```python
from build123d import *

# Parameters (mm, degrees)
SKETCH_1_W          = 550
SKETCH_1_H          = 550
SKETCH_1_R          = 200
EXTRUDE_1_DEPTH     = 3
SKETCH_2_R          = 2
CUT_EXTRUDE_1_DEPTH = 389.920300319
CHAMFER_1_SIZE      = 2


with BuildPart() as part:
    # 草图1 → 凸台-拉伸1 (new body)
    with BuildSketch(Plane(origin=(0, 0, 0), x_dir=(1, 0, 0), z_dir=(0, 1, 0))):
        Rectangle(SKETCH_1_W, SKETCH_1_H)
        with Locations(Location((0, 0, 0), (0, 0, 270))):
            Circle(SKETCH_1_R, mode=Mode.SUBTRACT)
    extrude(amount=EXTRUDE_1_DEPTH)

    # 草图2 → 切除-拉伸1 (cut, through all)
    with BuildSketch(Plane(origin=(0, 0, 0), x_dir=(1, 0, 0), z_dir=(0, 1, 0))):
        with Locations(Location((-260, 260, 0), (0, 0, 270))):
            Circle(SKETCH_2_R)
        with Locations(Location((-100, 260, 0), (0, 0, 270))):
            Circle(SKETCH_2_R)
        with Locations(Location((100, 260, 0), (0, 0, 90))):
            Circle(SKETCH_2_R)
        with Locations(Location((260, -100, 0), (0, 0, 90))):
            Circle(SKETCH_2_R)
        with Locations(Location((260, 100, 0), (0, 0, 270))):
            Circle(SKETCH_2_R)
        with Locations(Location((260, 260, 0), (0, 0, 270))):
            Circle(SKETCH_2_R)
        with Locations(Location((-100, -260, 0), (0, 0, 90))):
            Circle(SKETCH_2_R)
        with Locations(Location((100, -260, 0), (0, 0, 270))):
            Circle(SKETCH_2_R)
        with Locations(Location((260, -260, 0), (0, 0, 270))):
            Circle(SKETCH_2_R)
        with Locations(Location((-260, 100, 0), (0, 0, 90))):
            Circle(SKETCH_2_R)
        with Locations(Location((-260, -100, 0), (0, 0, 270))):
            Circle(SKETCH_2_R)
        with Locations(Location((-260, -260, 0), (0, 0, 270))):
            Circle(SKETCH_2_R)
    extrude(amount=CUT_EXTRUDE_1_DEPTH, mode=Mode.SUBTRACT)

    # 倒角1
    chamfer_1_edges = [part.edges().sort_by_distance(p)[0] for p in [
        (-260, 3, -98),
        (-260, 3, 98),
        (-260, 3, 258),
        (-100, 3, 262),
        (100, 3, 258),
        (260, 3, 258),
        (260, 3, 102),
        (260, 3, -102),
        (260, 0, -262),
        (100, 3, -258),
        (-100, 3, -262),
        (-260, 3, -262),
    ]]
    chamfer(chamfer_1_edges, length=CHAMFER_1_SIZE)


solid = part.part
```
Source: CAD feature listing. Evaluate the final solid. Frame: model axes, mm. Give positions to 0.01 mm unless a question says otherwise; leave off trailing zeros. Loops run counter-clockwise (first coordinate to the right, second up) from the corner with the lowest first, then second, coordinate; pieces in that order, holes last. Notation, with made-up numbers: (27, 15) -> (80, 15) arc R21 ccw to (80, 22) -> close; hole circle Ø5 at (76, 28.5). An arc over 180 degrees is marked (long way). Put each result on its own line as item: value. Start each with the question number.
1) Draft query along X for faces 1 (the face through (118, 3, -187)), 2 (the face through (60.075, 1.479, 190.764)). Return one class per face: released by +X, released by -X, zero draft, split by the parting line, or undercut.
2) Contact query for flat-ended pins moving along their axis: P1, Ø5, axis at x = 260, z = 260, coming from the -Y side; P2, Ø3, axis at x = 100, z = 260, coming from the +Y side; P3, Ø4.5, axis at x = 100, z = -260, coming from the +Y side; P4, Ø6.5, axis at x = -100, z = -260, coming from the +Y side. Output: stop coordinate, or through.
3) Cut plane A-A (x = 0). Return loops of the section in (y, z), then the cut area to 3 significant figures.
4) Cut plane C-C (y = 0.45). State how many separate pieces and enclosed holes the cut face has, then the cut area to 3 significant figures.
5) Material intervals for probe 1 along Z at (x, y) = (-260, 0.3); probe 2 along X at (y, z) = (0.7, -260), sorted ascending.
6) Cut plane B-B (z = 0). Return loops of the section in (x, y).
Results are:
1. face 1: zero draft
1. face 2: undercut
2. P1: stops at y = 0
2. P2: passes through
2. P3: stops at y = 1.25
2. P4: stops at y = 2.25
3. outline: (0, -275) -> (3, -275) -> (3, -200) -> (0, -200) -> close; (0, 200) -> (3, 200) -> (3, 275) -> (0, 275) -> close
3. area: 450 mm2
4. separate pieces: 1
4. enclosed holes: 13
4. area: 177,000 mm2
5. probe 1: z = -275 to -262, -258 to -102, -98 to 98, 102 to 258, 262 to 275
5. probe 2: x = -275 to -262, -258 to -102, -98 to 98, 102 to 256.7, 263.3 to 275
6. outline: (-275, 0) -> (-200, 0) -> (-200, 3) -> (-275, 3) -> close; (200, 0) -> (275, 0) -> (275, 3) -> (200, 3) -> close
